Model file for the job. Use its own axes, mm. A direction names the side the tool comes from. Round coordinates to 2 decimals unless told otherwise and drop trailing zeros. Order: outer loops, then holes, each group sorted by start corner. A loop starts at its lowest first (then second) coordinate and runs counter-clockwise, first axis right, second up. Notation, with made-up numbers: (69, -12) - (111, -12) arc R15 ccw to (111, 16) - close; hole circle Ø10 at (28.25, 2.5). An arc over 180 degrees is marked (long way). Put each result on its own line as item: value. Start each with the question number.
Item 1: Mould opens along Z. For faces 1 (the face through (5.987, -0.776, -4.697)), 2 (the face through (0, -1, -6.336)), 3 (the face through (-3.25, 2, -4)) say: pulls with the +Z half, pulls with the -Z half, needs draft (parallel to the pull), parting line crosses it, or undercut.
Item 2: Saw through at B-B on y = -0.4. List the corners of the cut face in (x, z), plus the area to 3 significant figures.
Item 3: Saw through at D-D on z = 0.25. List the corners of the cut face in (x, y).
Item 4: Probe probe 1 along X at (y, z) = (2, -1.5); probe 2 along Y at (x, z) = (0.5, 2.25); probe 3 along X at (y, z) = (-1.05, -3). List the from-to ranges inside material, lowest first.
Item 5: Saw through at C-C on x = 2.5. List the corners of the cut face in (y, z).
Item 6: Which spindle directions (+Z, -Z, +X, -X, +Y, -Y) get a long thin tool onto all of the face, cutting with end or side? Do faces 4 (the face through (3.25, 2, -4)), 5 (the face through (0, 2, -6.255)), 6 (the face through (5.232, -0.776, 6.995)), 7 (the face through (0, -1, 8.904)), 8 (the face through (0, 2, -1.255)). Say none if no direction does.
Item 7: Pin check, flat tips, straight feed: pin 1 Ø1.6 at (y, z) = (2, -4) entering from -X; pin 2 Ø2.5 at (x, z) = (5.52, -3.8) entering from +Y; pin 3 Ø2.5 at (x, y) = (-0.5, 1.5) entering from -Z. Stop position of each tip, or through.
Item 8: Saw through at A-A on x = 5. List the corners of the cut face in (y, z).
```python
from build123d import *

# Parameters (mm, degrees)
F0_R     = 1.016
F1_DEPTH = 1.5748
F2_W     = 6.5
F2_H     = 5
F3_DEPTH = 3.2


with BuildPart() as f1:
    # F0 (on Front) → F1 (new body)
    with BuildSketch(Plane.XZ):
        with BuildLine():
            Line((0.692302, 8.904484), (-0.577698, 8.904484))
            ThreePointArc((-0.577698, 8.904484), (-5.067826, 7.044612), (-6.927698, 2.554484))
            Line((-6.927698, 2.554484), (-6.927698, -6.335516))
            Line((-6.927698, -6.335516), (7.042302, -6.335516))
            Line((7.042302, -6.335516), (7.042302, 2.554484))
            ThreePointArc((7.042302, 2.554484), (5.18243, 7.044612), (0.692302, 8.904484))
        make_face()
        with Locations((-5.403698, -3.795516)):
            Circle(F0_R, mode=Mode.SUBTRACT)
        with Locations((5.518302, -3.795516)):
            Circle(F0_R, mode=Mode.SUBTRACT)
    extrude(amount=F1_DEPTH)

    # F2 (on face) → F3 (join)
    with BuildSketch(Plane.XZ):
        with Locations((0, -3.755355)):
            Rectangle(F2_W, F2_H)
    extrude(amount=-F3_DEPTH)


solid = f1.part
```
Results found:
1. face 1: undercut
1. face 2: pulls with the -Z half
1. face 3: needs draft
2. outline: (-6.93, -6.34) - (7.04, -6.34) - (7.04, 2.55) arc R6.35 ccw to (0.69, 8.9) - (-0.58, 8.9) arc R6.35 ccw to (-6.93, 2.55) - close; hole circle Ø2.03 at (-5.4, -3.8); hole circle Ø2.03 at (5.52, -3.8)
2. area: 189 mm²
3. outline: (-6.93, -1.57) - (7.04, -1.57) - (7.04, 0) - (-6.93, 0) - close
4. probe 1: x = -3.25 to 3.25
4. probe 2: y = -1.57 to 0
4. probe 3: x = -6.93 to -6.04, -4.77 to 4.89, 6.15 to 7.04
5. outline: (-1.57, -6.34) - (0, -6.34) - (0, -6.26) - (3.2, -6.26) - (3.2, -1.26) - (0, -1.26) - (0, 8.64) - (-1.57, 8.64) - close
6. face 4: +Z, -Z, +X, +Y
6. face 5: -Z, +X, -X, +Y
6. face 6: +Z, +X, +Y, -Y
6. face 7: +Z, +X, -X, +Y, -Y
6. face 8: +Z, +X, -X, +Y
7. pin 1: stops at x = -3.25
7. pin 2: stops at y = 0
7. pin 3: stops at z = -6.26
8. outline: (-1.57, -6.34) - (0, -6.34) - (0, -4.67) - (-1.57, -4.67) - close; (-1.57, -2.92) - (0, -2.92) - (0, 7.22) - (-1.57, 7.22) - close
